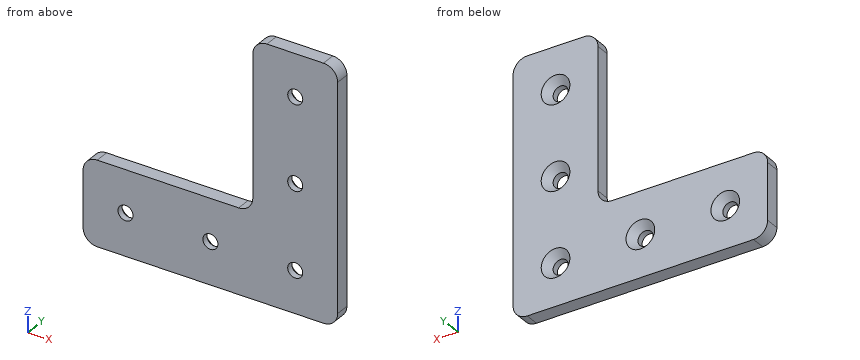
Autodesk Inventor part; units mm, degrees
ref_plane "YZ Plane" through (0, 0, 0) normal (1, 0, 0) x (0, 1, 0)
ref_plane "XZ Plane" through (0, 0, 0) normal (0, 1, 0) x (-1, 0, 0)
ref_plane "XY Plane" through (0, 0, 0) normal (0, 0, 1) x (1, 0, 0)
sketch "Sketch1" plane through (0, 0, 0) normal (0, 1, 0) x (-1, 0, 0)
  line L0 (0, 0) -> (19.05, 0)
  line L1 (38.1, 38.1) -> (38.1, 114.3)
  line L2 (38.1, 114.3) -> (0, 114.3)
  line L3 (0, 114.3) -> (0, 0)
  line L4 (0, 0) -> (114.3, 0)
  line L5 (114.3, 0) -> (114.3, 38.1)
  line L6 (114.3, 38.1) -> (38.1, 38.1)
  line L7 (0, 38.1) -> (0, 0)
  line L8 (19.05, 114.3) -> (19.05, 19.05) construction
  line L9 (19.05, 19.05) -> (114.3, 19.05) construction
  point P0 (19.05, 95.25)
  point P1 (19.05, 57.15)
  point P2 (57.15, 19.05)
  point P3 (95.25, 19.05)
  dimension "d3" = 38.1
  dimension "d4" = 114.3
  dimension "d5" = 114.3
  dimension "d6" = 38.1
  dimension "d9" = 19.05
  dimension "d10" = 19.05
  dimension "d11" = 19.05
  dimension "d12" = 57.15
  dimension "d13" = 19.05
  dimension "d14" = 57.15
extrude "Extrusion1" add sketch "Sketch1" against normal blind 6.35
hole "Hole1" at (-19.05, 0, 95.25) at (-19.05, 0, 57.15) at (-57.15, 0, 19.05) at (-95.25, 0, 19.05) at (-19.05, 0, 19.05) direction (0, -1, 0) diameter 6.7564 end through all countersink diameter 12.8778 countersink angle 82
fillet "Fillet1" radius 6.35 6 edges at (0, -3.175, 114.3) (0, -3.175, 0) (-38.1, -3.175, 114.3) (-38.1, -3.175, 38.1) (-114.3, -3.175, 0) (-114.3, -3.175, 38.1)
equation "\"d3\" = d6"
equation "\"d4\" = d5"
equation "\"d9\" = d10"
properties part number "angle-90-plate" material "Aluminum 6061"
Geometry: final body of the model. Coordinates: model frame, mm. Give positions to 0.01 mm unless a question says otherwise; leave off trailing zeros. Write each loop counter-clockwise with the first axis right and the second up, starting at its lowest first coordinate (ties: lowest second). Pieces come first, ordered by that corner, then holes. Notation, with made-up numbers: (38, 87) -> (60, 87) arc R27 cw to (60, 124) -> close; hole circle Ø2 at (55, 49). An arc over 180 degrees is marked (long way). Answer in a Markdown table with one row per item.
(1) Ray query, line 1 along Z through (x, y) = (-19.05, -4.6); line 2 along X through (y, z) = (-4.9, 19.05); line 3 along Z through (x, y) = (-15.5, -1.75). Return the intervals inside material, ascending. Write a range as [from, to].
Answers below:
| item | result |
|---|---|
| line 1 | [0, 15.67], [22.43, 53.77], [60.53, 91.87], [98.63, 114.3] |
| line 2 | [-114.3, -98.63], [-91.87, -60.53], [-53.77, -22.43], [-15.67, 0] |
| line 3 | [0, 15.65], [22.45, 53.75], [60.55, 91.85], [98.65, 114.3] |
(2) Section query A-A on z = 19.05. Return loops of the section in (x, y), then the cut area to 3 significant figures.
Answers below:
| item | result |
|---|---|
| outline | (-114.3, -6.35) -> (-98.63, -6.35) -> (-98.63, -3.52) -> (-101.69, 0) -> (-114.3, 0) -> close; (-91.87, -6.35) -> (-60.53, -6.35) -> (-60.53, -3.52) -> (-63.59, 0) -> (-88.81, 0) -> (-91.87, -3.52) -> close; (-53.77, -6.35) -> (-22.43, -6.35) -> (-22.43, -3.52) -> (-25.49, 0) -> (-50.71, 0) -> (-53.77, -3.52) -> close; (-15.67, -6.35) -> (0, -6.35) -> (0, 0) -> (-12.61, 0) -> (-15.67, -3.52) -> close |
| area | 565 mm^2 |
(3) Section query B-B on x = -19.05. Return loops of the section in (y, z), then the cut area to 3 significant figures.
Answers below:
| item | result |
|---|---|
| outline | (-6.35, 0) -> (0, 0) -> (0, 12.61) -> (-3.52, 15.67) -> (-6.35, 15.67) -> close; (-6.35, 22.43) -> (-3.52, 22.43) -> (0, 25.49) -> (0, 50.71) -> (-3.52, 53.77) -> (-6.35, 53.77) -> close; (-6.35, 60.53) -> (-3.52, 60.53) -> (0, 63.59) -> (0, 88.81) -> (-3.52, 91.87) -> (-6.35, 91.87) -> close; (-6.35, 98.63) -> (-3.52, 98.63) -> (0, 101.69) -> (0, 114.3) -> (-6.35, 114.3) -> close |
| area | 565 mm^2 |
(4) Section query C-C on y = -5.25. Return loops of the section in (x, z), then the cut area to 3 significant figures.
Answers below:
| item | result |
|---|---|
| outline | (-114.3, 6.35) arc R6.35 ccw to (-107.95, 0) -> (-6.35, 0) arc R6.35 ccw to (0, 6.35) -> (0, 107.95) arc R6.35 ccw to (-6.35, 114.3) -> (-31.75, 114.3) arc R6.35 ccw to (-38.1, 107.95) -> (-38.1, 44.45) arc R6.35 cw to (-44.45, 38.1) -> (-107.95, 38.1) arc R6.35 ccw to (-114.3, 31.75) -> close; hole circle Ø6.76 at (-95.25, 19.05); hole circle Ø6.76 at (-57.15, 19.05); hole circle Ø6.76 at (-19.05, 19.05); hole circle Ø6.76 at (-19.05, 57.15); hole circle Ø6.76 at (-19.05, 95.25) |
| area | 7,040 mm^2 |
(5) Section query D-D on x = -57.15. Return loops of the section in (y, z).
Answers below:
| item | result |
|---|---|
| outline | (-6.35, 0) -> (0, 0) -> (0, 12.61) -> (-3.52, 15.67) -> (-6.35, 15.67) -> close; (-6.35, 22.43) -> (-3.52, 22.43) -> (0, 25.49) -> (0, 38.1) -> (-6.35, 38.1) -> close |
(6) Pin query (flat end, axial travel): pin 1 (2 mm diameter, centred on y = -1.5, z = 52.5, fed in from +X); pin 2 (1.9 mm diameter, centred on y = -3.5, z = 65, fed in from -X); pin 3 (5.5 mm diameter, centred on x = -19.05, z = 57.15, fed in from -Y); pin 4 (9 mm diameter, centred on x = -95.25, z = 19.05, fed in from +Y). Return the tip coordinate at first contact, or that it passes through.
Answers below:
| item | result |
|---|---|
| pin 1 | x = 0 |
| pin 2 | x = -38.1 |
| pin 3 | through |
| pin 4 | y = -2.23 |
